Can you work these out from the model? Positions are in its coordinate system, mm. Face numbers are marked on the shaded views. A direction names the side the tool comes from. Round coordinates to 2 decimals unless told otherwise and drop trailing zeros. Loops run counter-clockwise (first coordinate to the right, second up) from the corner with the lowest first, then second, coordinate; pieces in that order, holes last.
(1) If I drill on line 1 along X through (y, z) = (4, 6); line 2 along Z through (x, y) = (-1, -16), over which ranges is the centre line in solid material (lowest first)?
(2) Thinking about a two-plate mould opening in Y: for the marked faces 4, 5 and 6, which applies, released by +Y, released by -Y, zero draft, split by the parting line, or undercut?
(3) Will these pins go through, and if not, where does the flat tip stop? pin 1 Ø1.6 at (x, z) = (-7.5, -20.5) entering from +Y; pin 2 Ø3 at (y, z) = (0, 25.25) entering from +X; pin 3 Ø24.5 at (x, y) = (11.5, -5) entering from -Z; pin 4 Ø1.7 at (x, z) = (25, 0.5) entering from +Y.
(4) I want a section at B-B on y = -15. Write out the boundary of the cut face in (x, z), plus the area to 3 significant figures.
(5) Which directions (+Z, -Z, +X, -X, +Y, -Y) give clear straight access to the entire face, cutting with the end or side of a thin tool? Please do the marked faces 1, 2 and 3.
(6) I want a section at C-C on x = 22.5. Write out the boundary of the cut face in (y, z).
(7) I want a section at A-A on y = 7.5. Write out the boundary of the cut face in (x, z), plus the area to 3 significant figures.
from build123d import *

# Parameters (mm, degrees)
SKETCH_1_W                         = 50
SKETCH_1_H                         = 50
SKETCH_1_R                         = 16
SM_BASE_FLANGE_1_DEPTH             = 1
SM_EDGE_FLANGE_1_STRIP_W           = 5.4732
SM_EDGE_FLANGE_1_STRIP_H           = 1
SM_EDGE_FLANGE_1_STRIP_CUT_DEPTH   = 50
SM_EDGE_FLANGE_1_STRIP_2_W         = 5.4732
SM_EDGE_FLANGE_1_STRIP_2_H         = 1
SM_EDGE_FLANGE_1_STRIP_CUT_2_DEPTH = 50
SM_EDGE_FLANGE_1_DEPTH             = 50
SM_EDGE_FLANGE_1_BEND_DEPTH        = 50
SM_EDGE_FLANGE_2_STRIP_W           = 5.4732
SM_EDGE_FLANGE_2_STRIP_H           = 1
SM_EDGE_FLANGE_2_STRIP_CUT_DEPTH   = 48.5268
SM_EDGE_FLANGE_2_STRIP_2_W         = 5.4732
SM_EDGE_FLANGE_2_STRIP_2_H         = 1
SM_EDGE_FLANGE_2_STRIP_CUT_2_DEPTH = 48.5268
SM_EDGE_FLANGE_2_DEPTH             = 48.5268
SM_EDGE_FLANGE_2_BEND_DEPTH        = 48.5268
SKETCH_23_R                        = 1
CUT_EXTRUDE_1_DEPTH                = 98
CUT_EXTRUDE_3_REACH                = 67.886
SKETCH_27_R                        = 3.5
SKETCH_27_R_2                      = 1
EXTRUDE_START                      = -1
SKETCH_30_R                        = 3.5
SKETCH_30_R_2                      = 1.5
EXTRUDE_1_DEPTH                    = 1
SKETCH_33_R                        = 3.5
EXTRUDE_2_DEPTH                    = 1
SKETCH_36_R                        = 1.5
CUT_EXTRUDE_4_DEPTH                = 1


# Sheet-metal steps are written as plain solids
with BuildPart() as part:
    # Sketch 1 → 基材-凸緣1 (new body)
    with BuildSketch(Plane.XY):
        Rectangle(SKETCH_1_W, SKETCH_1_H)
        Circle(SKETCH_1_R, mode=Mode.SUBTRACT)
    extrude(amount=-SM_BASE_FLANGE_1_DEPTH)

    # 邊線-凸緣1 strip (across the edge) → 邊線-凸緣1 strip cut (cut)
    with BuildSketch(Plane(origin=(-25, 25, -1), x_dir=(0, -1, 0), z_dir=(1, 0, 0))):
        with Locations((-2, -0.5)):
            Rectangle(SM_EDGE_FLANGE_1_STRIP_W, SM_EDGE_FLANGE_1_STRIP_H)
    extrude(amount=SM_EDGE_FLANGE_1_STRIP_CUT_DEPTH, mode=Mode.SUBTRACT)

    # 邊線-凸緣1 strip 2 (across the edge) → 邊線-凸緣1 strip cut 2 (cut)
    with BuildSketch(Plane(origin=(25, -25, -1), x_dir=(0, 1, 0), z_dir=(-1, 0, 0))):
        with Locations((-2, -0.5)):
            Rectangle(SM_EDGE_FLANGE_1_STRIP_2_W, SM_EDGE_FLANGE_1_STRIP_2_H)
    extrude(amount=SM_EDGE_FLANGE_1_STRIP_CUT_2_DEPTH, mode=Mode.SUBTRACT)

    # 邊線-凸緣1 section (across the edge) → 邊線-凸緣1 (add)
    with BuildSketch(Plane(origin=(-25, 25, -1), x_dir=(0, -1, 0), z_dir=(1, 0, 0))):
        with BuildLine():
            Line((-1, 0.7366), (-1, 30))
            Line((-1, 30), (0, 30))
            Line((0, 30), (0, 0.7366))
            ThreePointArc((0, 0.7366), (0.215745145, 0.215745145), (0.7366, 0))
            Line((0.7366, 0), (0.7366, -1))
            ThreePointArc((0.7366, -1), (-0.491361636, -0.491361636), (-1, 0.7366))
        make_face()
    extrude(amount=SM_EDGE_FLANGE_1_DEPTH)

    # 邊線-凸緣1 section 2 (across the edge) → 邊線-凸緣1 bend (add)
    with BuildSketch(Plane(origin=(25, -25, -1), x_dir=(0, 1, 0), z_dir=(-1, 0, 0))):
        with BuildLine():
            Line((-1, 0.7366), (-1, 30))
            Line((-1, 30), (0, 30))
            Line((0, 30), (0, 0.7366))
            ThreePointArc((0, 0.7366), (0.215745145, 0.215745145), (0.7366, 0))
            Line((0.7366, 0), (0.7366, -1))
            ThreePointArc((0.7366, -1), (-0.491361636, -0.491361636), (-1, 0.7366))
        make_face()
    extrude(amount=SM_EDGE_FLANGE_1_BEND_DEPTH)

    # 邊線-凸緣2 strip (across the edge) → 邊線-凸緣2 strip cut (cut)
    with BuildSketch(Plane(origin=(25, -24.2634, 0), x_dir=(-1, 0, 0), z_dir=(0, 1, 0))):
        with Locations((-2, -0.5)):
            Rectangle(SM_EDGE_FLANGE_2_STRIP_W, SM_EDGE_FLANGE_2_STRIP_H)
    extrude(amount=SM_EDGE_FLANGE_2_STRIP_CUT_DEPTH, mode=Mode.SUBTRACT)

    # 邊線-凸緣2 strip 2 (across the edge) → 邊線-凸緣2 strip cut 2 (cut)
    with BuildSketch(Plane(origin=(-25, 24.2634, 0), x_dir=(1, 0, 0), z_dir=(0, -1, 0))):
        with Locations((-2, -0.5)):
            Rectangle(SM_EDGE_FLANGE_2_STRIP_2_W, SM_EDGE_FLANGE_2_STRIP_2_H)
    extrude(amount=SM_EDGE_FLANGE_2_STRIP_CUT_2_DEPTH, mode=Mode.SUBTRACT)

    # 邊線-凸緣2 section (across the edge) → 邊線-凸緣2 (add)
    with BuildSketch(Plane(origin=(25, -24.2634, 0), x_dir=(-1, 0, 0), z_dir=(0, 1, 0))):
        with BuildLine():
            Line((-1, 0.7366), (-1, 30))
            Line((-1, 30), (0, 30))
            Line((0, 30), (0, 0.7366))
            ThreePointArc((0, 0.7366), (0.215745145, 0.215745145), (0.7366, 0))
            Line((0.7366, 0), (0.7366, -1))
            ThreePointArc((0.7366, -1), (-0.491361636, -0.491361636), (-1, 0.7366))
        make_face()
    extrude(amount=SM_EDGE_FLANGE_2_DEPTH)

    # 邊線-凸緣2 section 2 (across the edge) → 邊線-凸緣2 bend (add)
    with BuildSketch(Plane(origin=(-25, 24.2634, 0), x_dir=(1, 0, 0), z_dir=(0, -1, 0))):
        with BuildLine():
            Line((-1, 0.7366), (-1, 30))
            Line((-1, 30), (0, 30))
            Line((0, 30), (0, 0.7366))
            ThreePointArc((0, 0.7366), (0.215745145, 0.215745145), (0.7366, 0))
            Line((0.7366, 0), (0.7366, -1))
            ThreePointArc((0.7366, -1), (-0.491361636, -0.491361636), (-1, 0.7366))
        make_face()
    extrude(amount=SM_EDGE_FLANGE_2_BEND_DEPTH)

    # 草圖23 → 除料-伸長1 (cut)
    with BuildSketch(Plane(origin=(0, 26, 0), x_dir=(1, 0, 0), z_dir=(0, 1, 0))):
        with BuildLine():
            Line((25, 31), (0, 31))
            ThreePointArc((0, 31), (4.971280899, 29.748587256), (8.757585745, 26.292641186))
            Line((8.757585745, 26.292641186), (25, 1.7366))
            Line((25, 1.7366), (25, 31))
        make_face()
        with BuildLine():
            ThreePointArc((-8.757585745, 26.292641186), (-4.971280899, 29.748587256), (0, 31))
            Line((0, 31), (-25, 31))
            Line((-25, 31), (-25, 1.7366))
            Line((-25, 1.7366), (-8.757585745, 26.292641186))
        make_face()
        with BuildLine():
            ThreePointArc((1, 28), (0.707106781, 28.707106781), (0, 29))
            Line((0, 29), (0, 27))
            ThreePointArc((0, 27), (0.707106781, 27.292893219), (1, 28))
        make_face()
        with BuildLine():
            Line((0, 27), (0, 29))
            ThreePointArc((0, 29), (-1, 28), (0, 27))
        make_face()
        with Locations(Location((-7.5, 20.5, 0), (0, 0, 90))):
            Circle(SKETCH_23_R)
        with Locations(Location((7.5, 20.5, 0), (0, 0, 90))):
            Circle(SKETCH_23_R)
        with BuildLine():
            ThreePointArc((1, 13), (0.707106781, 13.707106781), (0, 14))
            Line((0, 14), (0, 12))
            ThreePointArc((0, 12), (0.707106781, 12.292893219), (1, 13))
        make_face()
        with BuildLine():
            Line((0, 12), (0, 14))
            ThreePointArc((0, 14), (-1, 13), (0, 12))
        make_face()
        with BuildLine():
            ThreePointArc((3.5, 20.5), (2.474873734, 22.974873734), (0, 24))
            Line((0, 24), (0, 17))
            ThreePointArc((0, 17), (2.474873734, 18.025126266), (3.5, 20.5))
        make_face()
        with BuildLine():
            Line((0, 17), (0, 24))
            ThreePointArc((0, 24), (-3.5, 20.5), (0, 17))
        make_face()
    extrude(amount=-CUT_EXTRUDE_1_DEPTH, mode=Mode.SUBTRACT)

    # 除料-伸長3: up to this face of the body (flat: up to its plane)
    cut_extrude_3_end = Plane(part.part.faces().sort_by_distance((-26, 0, 15.3683))[0])
    # 草圖27 → 除料-伸長3 (cut, up to the picked face)
    with BuildSketch(Plane(origin=(26, 0, 0), x_dir=(0, 0, -1), z_dir=(1, 0, 0)), mode=Mode.PRIVATE) as cut_extrude_3_sk1:
        with BuildLine():
            Line((-30, -24.2634), (-0.7366, -24.2634))
            Line((-0.7366, -24.2634), (-23.651269893, -8.68300712))
            ThreePointArc((-23.651269893, -8.68300712), (-28.24742476, 0), (-23.651269893, 8.68300712))
            Line((-23.651269893, 8.68300712), (-0.7366, 24.2634))
            Line((-0.7366, 24.2634), (-30, 24.2634))
            Line((-30, 24.2634), (-30, -24.2634))
        make_face()
    cut_extrude_3_tool1 = split(extrude(cut_extrude_3_sk1.sketch, amount=-CUT_EXTRUDE_3_REACH, mode=Mode.PRIVATE), bisect_by=cut_extrude_3_end, keep=Keep.BOTH, mode=Mode.PRIVATE)
    # 草圖27 → 除料-伸長3 (cut, up to the picked face)
    with BuildSketch(Plane(origin=(26, 0, 0), x_dir=(0, 0, -1), z_dir=(1, 0, 0)), mode=Mode.PRIVATE) as cut_extrude_3_sk2:
        with Locations(Location((-17.74742476, 0, 0), (0, 0, 180))):
            Circle(SKETCH_27_R)
    cut_extrude_3_tool2 = split(extrude(cut_extrude_3_sk2.sketch, amount=-CUT_EXTRUDE_3_REACH, mode=Mode.PRIVATE), bisect_by=cut_extrude_3_end, keep=Keep.BOTH, mode=Mode.PRIVATE)
    # 草圖27 → 除料-伸長3 (cut, up to the picked face)
    with BuildSketch(Plane(origin=(26, 0, 0), x_dir=(0, 0, -1), z_dir=(1, 0, 0)), mode=Mode.PRIVATE) as cut_extrude_3_sk3:
        with Locations(Location((-17.74742476, -7.5, 0), (0, 0, 180))):
            Circle(SKETCH_27_R_2)
    cut_extrude_3_tool3 = split(extrude(cut_extrude_3_sk3.sketch, amount=-CUT_EXTRUDE_3_REACH, mode=Mode.PRIVATE), bisect_by=cut_extrude_3_end, keep=Keep.BOTH, mode=Mode.PRIVATE)
    # 草圖27 → 除料-伸長3 (cut, up to the picked face)
    with BuildSketch(Plane(origin=(26, 0, 0), x_dir=(0, 0, -1), z_dir=(1, 0, 0)), mode=Mode.PRIVATE) as cut_extrude_3_sk4:
        with Locations(Location((-25.24742476, 0, 0), (0, 0, 180))):
            Circle(SKETCH_27_R_2)
    cut_extrude_3_tool4 = split(extrude(cut_extrude_3_sk4.sketch, amount=-CUT_EXTRUDE_3_REACH, mode=Mode.PRIVATE), bisect_by=cut_extrude_3_end, keep=Keep.BOTH, mode=Mode.PRIVATE)
    # 草圖27 → 除料-伸長3 (cut, up to the picked face)
    with BuildSketch(Plane(origin=(26, 0, 0), x_dir=(0, 0, -1), z_dir=(1, 0, 0)), mode=Mode.PRIVATE) as cut_extrude_3_sk5:
        with Locations(Location((-17.74742476, 7.5, 0), (0, 0, 180))):
            Circle(SKETCH_27_R_2)
    cut_extrude_3_tool5 = split(extrude(cut_extrude_3_sk5.sketch, amount=-CUT_EXTRUDE_3_REACH, mode=Mode.PRIVATE), bisect_by=cut_extrude_3_end, keep=Keep.BOTH, mode=Mode.PRIVATE)
    # 草圖27 → 除料-伸長3 (cut, up to the picked face)
    with BuildSketch(Plane(origin=(26, 0, 0), x_dir=(0, 0, -1), z_dir=(1, 0, 0)), mode=Mode.PRIVATE) as cut_extrude_3_sk6:
        with Locations(Location((-10.24742476, 0, 0), (0, 0, 180))):
            Circle(SKETCH_27_R_2)
    cut_extrude_3_tool6 = split(extrude(cut_extrude_3_sk6.sketch, amount=-CUT_EXTRUDE_3_REACH, mode=Mode.PRIVATE), bisect_by=cut_extrude_3_end, keep=Keep.BOTH, mode=Mode.PRIVATE)
    add(cut_extrude_3_tool1.solids().sort_by(Axis((26, -23.696726, 15.3683), (-1, 0, 0)))[0], mode=Mode.SUBTRACT)
    add(cut_extrude_3_tool2.solids().sort_by(Axis((26, 0, 17.747425), (-1, 0, 0)))[0], mode=Mode.SUBTRACT)
    add(cut_extrude_3_tool3.solids().sort_by(Axis((26, -7.5, 17.747425), (-1, 0, 0)))[0], mode=Mode.SUBTRACT)
    add(cut_extrude_3_tool4.solids().sort_by(Axis((26, 0, 25.247425), (-1, 0, 0)))[0], mode=Mode.SUBTRACT)
    add(cut_extrude_3_tool5.solids().sort_by(Axis((26, 7.5, 17.747425), (-1, 0, 0)))[0], mode=Mode.SUBTRACT)
    add(cut_extrude_3_tool6.solids().sort_by(Axis((26, 0, 10.247425), (-1, 0, 0)))[0], mode=Mode.SUBTRACT)

    # 草圖30 → 填料-伸長1 (add)
    with BuildSketch(Plane.XZ.offset(26).offset(EXTRUDE_START)):
        with Locations(Location((0, -20.5, 0), (0, 0, 270))):
            Circle(SKETCH_30_R)
        with Locations(Location((0, -20.5, 0), (0, 0, 270))):
            Circle(SKETCH_30_R_2, mode=Mode.SUBTRACT)
    extrude(amount=EXTRUDE_1_DEPTH)

    # 草圖33 → 填料-伸長2 (add)
    with BuildSketch(Plane.ZY.offset(26).offset(EXTRUDE_START)):
        with Locations((17.74742476, 0)):
            Circle(SKETCH_33_R)
    extrude(amount=EXTRUDE_2_DEPTH)

    # 草圖36 → 除料-伸長4 (cut)
    with BuildSketch(Plane.ZY.offset(26)):
        with Locations((17.74742476, 0)):
            Circle(SKETCH_36_R)
    extrude(amount=-CUT_EXTRUDE_4_DEPTH, mode=Mode.SUBTRACT)


solid = part.part
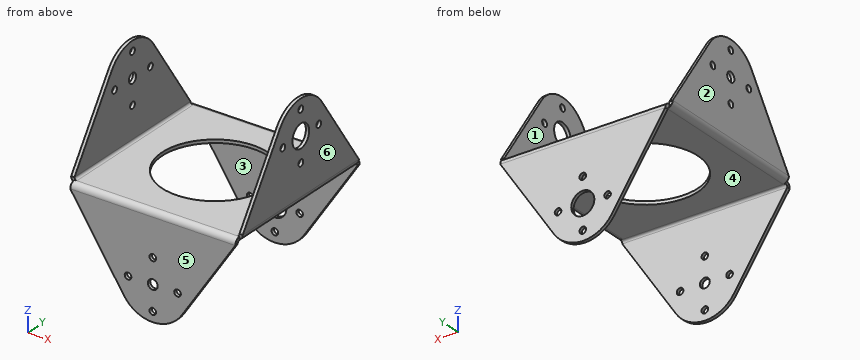
Filled sheet:
1. line 1: x = -26 to -25, 25 to 26
1. line 2: z = -1 to 0
2. face 4: undercut
2. face 5: released by -Y
2. face 6: zero draft
3. pin 1: passes through
3. pin 2: stops at x = 26
3. pin 3: stops at z = -1
3. pin 4: stops at y = 25.31
4. outline: (-26, 0.74) arc R1.74 ccw to (-24.26, -1) - (-5.57, -1) - (-5.57, 0) - (-24.26, 0) arc R0.74 cw to (-25, 0.74) - (-25, 14.36) - (-26, 14.36) - close; (5.57, -1) - (24.26, -1) arc R1.74 ccw to (26, 0.74) - (26, 14.36) - (25, 14.36) - (25, 0.74) arc R0.74 cw to (24.26, 0) - (5.57, 0) - close
4. area: 68.5 mm2
5. face 1: +Z, +Y, -Y
5. face 2: +Z, -Z, -X, +Y, -Y
5. face 3: -Z, +X, -X
6. outline: (-26, -5.52) - (-25, -5.52) - (-25, -1.74) arc R0.74 cw to (-24.26, -1) - (24.26, -1) arc R0.74 cw to (25, -1.74) - (25, -5.52) - (26, -5.52) - (26, -1.74) arc R1.74 ccw to (24.26, 0) - (-24.26, 0) arc R1.74 ccw to (-26, -1.74) - close
7. outline: (-26, 0.74) arc R1.74 ccw to (-24.26, -1) - (-14.13, -1) - (-14.13, 0) - (-24.26, 0) arc R0.74 cw to (-25, 0.74) - (-25, 16.75) - (-26, 16.75) - close; (-26, 18.75) - (-25, 18.75) - (-25, 25.1) - (-26, 25.1) - close; (14.13, -1) - (24.26, -1) arc R1.74 ccw to (26, 0.74) - (26, 16.75) - (25, 16.75) - (25, 0.74) arc R0.74 cw to (24.26, 0) - (14.13, 0) - close; (25, 18.75) - (26, 18.75) - (26, 25.1) - (25, 25.1) - close
7. area: 68.9 mm2
